Read the model definition and answer for the solid it produces. Units are mm, in the model's axes. Coordinates: 2 decimals unless noted, no trailing zeros. Loops run counter-clockwise (first coordinate to the right, second up) from the corner with the lowest first, then second, coordinate; pieces in that order, holes last.
Q1. Section D-D (y = 8.5) is taken. Give the vertices of the cut face in (x, z).
Q2. The mould has two halves that part along Z. Classify faces 1 (the face through (11.7, 2.46, -28.22)), 2 (the face through (-33.71, 7.41, 4.43)), 3 (the face through (11.7, 12.6, -28.22)), 4 (the face through (9.6, 0, -29.2)): pulls with the +Z half, pulls with the -Z half, needs draft (parallel to the pull), parting line crosses it, or undercut.
Q3. Flat-ended cylindrical pins translate along their axes: P1, Ø2, axis at y = 13.5, z = 20, coming from the +X side; P2, Ø2, axis at y = 13, z = -2, coming from the +X side; P3, Ø2, axis at y = 11, z = -27, coming from the -X side. Find the tip coordinate at first contact, or state that the pin passes through.
Q4. Section B-B (x = 0) is taken. Give the vertices of the cut face in (y, z).
Q5. Straight lines are drawn through the part: line 1 (X direction, y = 3.1, z = 0); line 2 (X direction, y = 1.25, z = 4); line 3 (Z direction, x = 15, y = 7). For each, find the intervals that lie inside material, in ascending order.
Q6. Section C-C (y = 12.5) is taken. Give the vertices of the cut face in (x, z), then the cut area to 3 significant figures.
Q7. Section A-A (z = 0) is taken. Give the vertices of the cut face in (x, y), then the cut area to 3 significant figures.
from build123d import *

# Parameters (mm, degrees)
FILLET1_R = 1


with BuildPart() as part:
    # Sketch1 → Revolve1 (revolve)
    with BuildSketch(Plane.XY, mode=Mode.PRIVATE) as revolve1_sk:
        with BuildLine():
            Line((-34, 0), (-30.55, 0))
            Line((-30.55, 0), (-30.55, 4.859058821))
            ThreePointArc((-30.55, 4.859058821), (-31.55625, 7.5), (-30.55, 10.140941179))
            Line((-30.55, 10.140941179), (-30.55, 15))
            Line((-30.55, 15), (-34, 15))
            Line((-34, 15), (-34, 0))
        make_face()
    revolve(revolve1_sk.sketch.rotate(Axis((0, 0, 0), (0, 1, 0)), 270), axis=Axis((0, 0, 0), (0, 1, 0)))

    # Fillet1
    fillet1_edges = [part.edges().sort_by_distance(p)[0] for p in [
        (0, 0, 34),
        (0, 15, 34),
    ]]
    fillet(fillet1_edges, radius=FILLET1_R)


solid = part.part
Numbers:
1. outline: circle Ø68 at (0, 0); hole circle Ø62.86 at (0, 0)
2. face 1: undercut
2. face 2: parting line crosses it
2. face 3: undercut
2. face 4: needs draft
3. P1: stops at x = 28.2
3. P2: stops at x = 33.99
3. P3: stops at x = -21.91
4. outline: (0, -33) arc R1 ccw to (1, -34) - (14, -34) arc R1 ccw to (15, -33) - (15, -30.55) - (10.14, -30.55) arc R3.97 cw to (4.86, -30.55) - (0, -30.55) - close; (0, 30.55) - (4.86, 30.55) arc R3.97 cw to (10.14, 30.55) - (15, 30.55) - (15, 33) arc R1 ccw to (14, 34) - (1, 34) arc R1 ccw to (0, 33) - close
5. line 1: x = -34 to -30.55, 30.55 to 34
5. line 2: x = -33.76 to -30.29, 30.29 to 33.76
5. line 3: z = -30.51 to -27.73, 27.73 to 30.51
6. outline: circle Ø68 at (0, 0); hole circle Ø61.1 at (0, 0)
6. area: 700 mm2
7. outline: (-34, 1) arc R1 ccw to (-33, 0) - (-30.55, 0) - (-30.55, 4.86) arc R3.97 cw to (-30.55, 10.14) - (-30.55, 15) - (-33, 15) arc R1 ccw to (-34, 14) - close; (30.55, 0) - (33, 0) arc R1 ccw to (34, 1) - (34, 14) arc R1 ccw to (33, 15) - (30.55, 15) - (30.55, 10.14) arc R3.97 cw to (30.55, 4.86) - close
7. area: 95.4 mm2
